Source: three-view drawing plus pictorial views. Frame: mm from the lowest corner of the part. Round coordinates to 2 decimals unless told otherwise and drop trailing zeros. Write each loop counter-clockwise with the first axis right and the second up, starting at its lowest first coordinate (ties: lowest second). Pieces come first, ordered by that corner, then holes. Notation, with made-up numbers: (16, -12) - (56, -12) arc R13 ccw to (56, -7) - close; hole circle Ø3 at (45, 34.5). An arc over 180 degrees is marked (long way). Write each question's results on one line, items separated by ' | '.
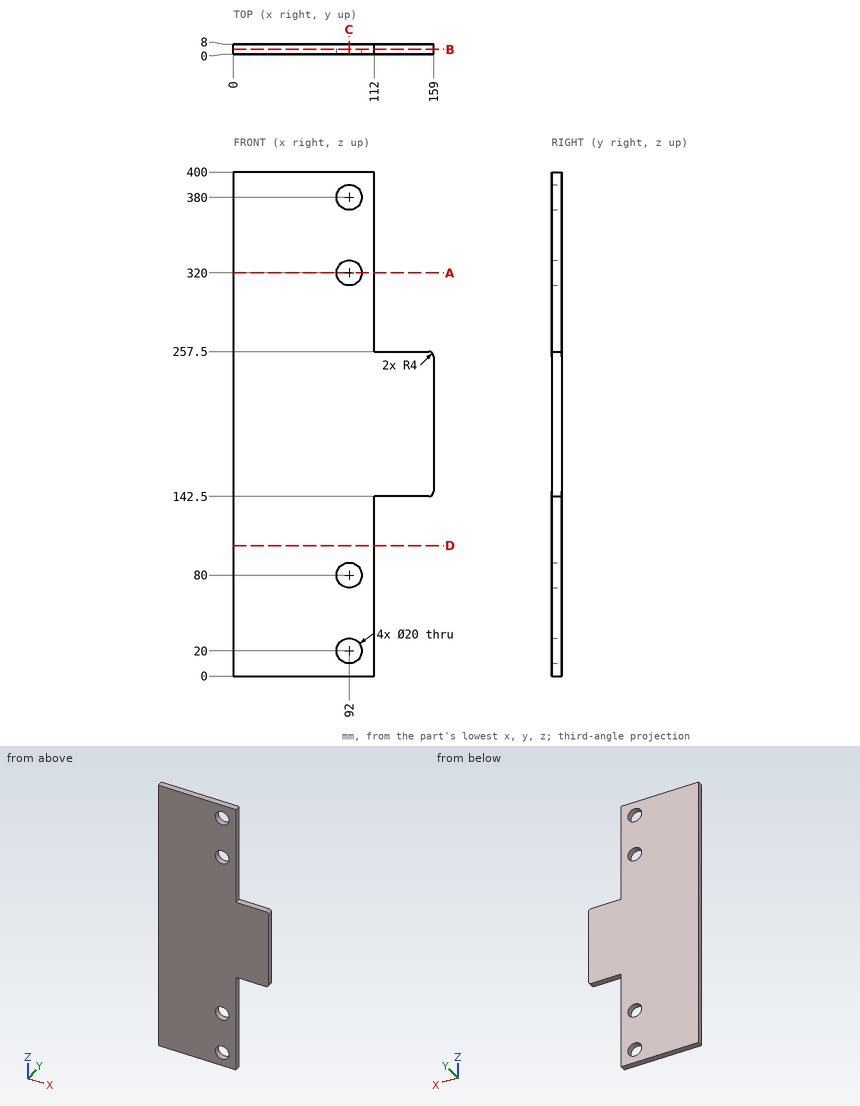
Q1. Section query A-A, the plane z = 320. Return loops of the section in (x, y), plus the area to 3 significant figures.
Answer block:
outline: (0, 0) - (82, 0) - (82, 8) - (0, 8) - close; (102, 0) - (112, 0) - (112, 8) - (102, 8) - close | area: 736 mm2
Q2. Section query D-D, the plane z = 103.5. Return loops of the section in (x, y), plus the area to 3 significant figures.
Answer block:
outline: (0, 0) - (112, 0) - (112, 8) - (0, 8) - close | area: 896 mm2
Q3. Pin query (flat end, axial travel): pin 1 (4 mm diameter, centred on x = 127.5, y = 4.5, fed in from -Z); pin 2 (4 mm diameter, centred on y = 4, z = 79.5, fed in from +X); pin 3 (3 mm diameter, centred on x = 114, y = 6, fed in from +Z). Return the tip coordinate at first contact, or that it passes through.
Answer block:
pin 1: z = 142.5 | pin 2: x = 112 | pin 3: z = 257.5
Q4. Section query B-B, the plane y = 3.75. Return loops of the section in (x, z), plus the area to 3 significant figures.
Answer block:
outline: (0, 0) - (112, 0) - (112, 142.5) - (155, 142.5) arc R4 ccw to (159, 146.5) - (159, 253.5) arc R4 ccw to (155, 257.5) - (112, 257.5) - (112, 400) - (0, 400) - close; hole circle Ø20 at (92, 20); hole circle Ø20 at (92, 80); hole circle Ø20 at (92, 320); hole circle Ø20 at (92, 380) | area: 48,900 mm2
Q5. Section query C-C, the plane x = 92. Return loops of the section in (y, z), plus the area to 3 significant figures.
Answer block:
outline: (0, 0) - (8, 0) - (8, 10) - (0, 10) - close; (0, 30) - (8, 30) - (8, 70) - (0, 70) - close; (0, 90) - (8, 90) - (8, 310) - (0, 310) - close; (0, 330) - (8, 330) - (8, 370) - (0, 370) - close; (0, 390) - (8, 390) - (8, 400) - (0, 400) - close | area: 2,560 mm2
Q6. Ray query, line 1 along Z through (x, y) = (92, 6); line 2 along X through (y, z) = (6, 80); line 3 along X through (y, z) = (3, 338.5). Return the intervals inside material, ascending.
Answer block:
line 1: 0 to 10, 30 to 70, 90 to 310, 330 to 370, 390 to 400 | line 2: 0 to 82, 102 to 112 | line 3: 0 to 112
